Source: CAD feature listing. Evaluate the final solid. Frame: model axes, mm. Coordinates: 2 decimals unless noted, no trailing zeros. Loops run counter-clockwise (first coordinate to the right, second up) from the corner with the lowest first, then second, coordinate; pieces in that order, holes last.
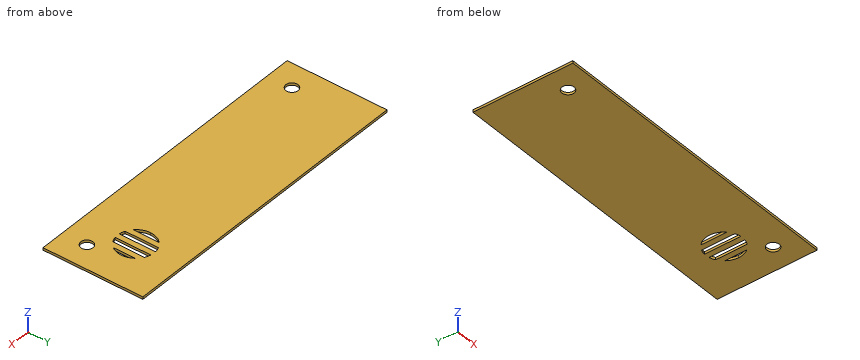
from build123d import *

# Parameters (mm, degrees)
SKETCH1_W           = 250
SKETCH1_H           = 82
BOSS_EXTRUDE1_DEPTH = 2
CUT_EXTRUDE1_DEPTH  = 3
SKETCH3_R           = 5
CUT_EXTRUDE2_DEPTH  = 3


with BuildPart() as part:
    # Sketch1 → Boss-Extrude1 (new body)
    with BuildSketch(Plane.XY):
        Rectangle(SKETCH1_W, SKETCH1_H)
    extrude(amount=BOSS_EXTRUDE1_DEPTH)

    # Sketch2 → Cut-Extrude1 (cut)
    with BuildSketch(Plane.XY.offset(2)):
        with BuildLine():
            ThreePointArc((74.195797737, 13.695923098), (70.866481051, 8.793255475), (69.695797737, 2.983780456))
            ThreePointArc((69.695797737, 2.983780456), (70.866481051, -2.825694564), (74.195797737, -7.728362187))
            Line((74.195797737, -7.728362187), (74.195797737, 13.695923098))
        make_face()
        with BuildLine():
            Line((83.195797737, 17.773650373), (82.193848931, 17.773650373))
            ThreePointArc((82.193848931, 17.773650373), (80.413006732, 17.359374398), (78.695797737, 16.73150754))
            Line((78.695797737, 16.73150754), (78.695797737, -10.763946629))
            ThreePointArc((78.695797737, -10.763946629), (80.899894424, -11.527977468), (83.195797737, -11.941031101))
            Line((83.195797737, -11.941031101), (83.195797737, 17.773650373))
        make_face()
        with BuildLine():
            ThreePointArc((92.195797737, 15.974161512), (90.014687146, 17.009093837), (87.695797737, 17.680718912))
            Line((87.695797737, 17.680718912), (87.695797737, -11.713158001))
            ThreePointArc((87.695797737, -11.713158001), (90.014687146, -11.041532926), (92.195797737, -10.006600601))
            Line((92.195797737, -10.006600601), (92.195797737, 15.974161512))
        make_face()
        with BuildLine():
            ThreePointArc((99.695797737, 2.983780456), (98.926047208, 7.727196946), (96.695797737, 11.983780456))
            Line((96.695797737, 11.983780456), (96.695797737, -6.016219544))
            ThreePointArc((96.695797737, -6.016219544), (98.926047208, -1.759636035), (99.695797737, 2.983780456))
        make_face()
    extrude(amount=-CUT_EXTRUDE1_DEPTH, mode=Mode.SUBTRACT)

    # Sketch3 → Cut-Extrude2 (cut)
    with BuildSketch(Plane.XY.offset(2)):
        with Locations((-105, -21)):
            Circle(SKETCH3_R)
        with Locations((105, -21)):
            Circle(SKETCH3_R)
    extrude(amount=-CUT_EXTRUDE2_DEPTH, mode=Mode.SUBTRACT)


solid = part.part
Q1. Section C-C, the plane x = -105. Return the cut outline in (y, z).
Q2. Section B-B, the plane z = 0.7. Return the cut outline in (x, y), plus the area to 3 significant figures.
Q3. Section D-D, the plane y = 6. Return the cut outline in (x, z), plus the area to 3 significant figures.
Q4. Contact query for a flat-ended pin moving along its axis: pin 1 Ø8 at (x, y) = (25, 32.5) entering from -Z. Output: stop coordinate, or through.
Q5. Line query: line 1 along Y through (x, z) = (105, 0.55); line 2 along X through (y, z) = (1, 0.25); line 3 along X through (y, z) = (10, 1). Output: solid intervals per line, ascending.
Q6. Section A-A, the plane y = -21. Return the cut outline in (x, z).
Derived:
1. outline: (-41, 0) - (-26, 0) - (-26, 2) - (-41, 2) - close; (-16, 0) - (41, 0) - (41, 2) - (-16, 2) - close
2. outline: (-125, -41) - (125, -41) - (125, 41) - (-125, 41) - close; hole circle Ø10 at (-105, -21); hole (74.2, -7.73) - (74.2, 13.7) arc R15 ccw to start; hole (78.7, -10.76) arc R15 ccw to (83.2, -11.94) - (83.2, 17.77) - (82.19, 17.77) arc R15 ccw to (78.7, 16.73) - close; hole (87.7, -11.71) arc R15 ccw to (92.2, -10.01) - (92.2, 15.97) arc R15 ccw to (87.7, 17.68) - close; hole (96.7, -6.02) arc R15 ccw to (96.7, 11.98) - close; hole circle Ø10 at (105, -21)
2. area: 20,000 mm2
3. outline: (-125, 0) - (70, 0) - (70, 2) - (-125, 2) - close; (74.2, 0) - (78.7, 0) - (78.7, 2) - (74.2, 2) - close; (83.2, 0) - (87.7, 0) - (87.7, 2) - (83.2, 2) - close; (92.2, 0) - (96.7, 0) - (96.7, 2) - (92.2, 2) - close; (99.39, 0) - (125, 0) - (125, 2) - (99.39, 2) - close
3. area: 468 mm2
4. pin 1: stops at z = 0
5. line 1: y = -41 to -26, -16 to 41
5. line 2: x = -125 to 69.83, 74.2 to 78.7, 83.2 to 87.7, 92.2 to 96.7, 99.56 to 125
5. line 3: x = -125 to 71.44, 74.2 to 78.7, 83.2 to 87.7, 92.2 to 96.7, 97.95 to 125
6. outline: (-125, 0) - (-110, 0) - (-110, 2) - (-125, 2) - close; (-100, 0) - (100, 0) - (100, 2) - (-100, 2) - close; (110, 0) - (125, 0) - (125, 2) - (110, 2) - close
